from build123d import *

# Parameters (mm, degrees)
SKETCH_1_W                  = 325
SKETCH_1_H                  = 205
EXTRUDE_1_DEPTH             = 14
SKETCH_2_W                  = 7
SKETCH_2_H                  = 130
CUT_EXTRUDE_1_DEPTH         = 341.852240714
CUT_EXTRUDE_2_DEPTH         = 10
SKETCH_4_W                  = 3
SKETCH_4_H                  = 6
CUT_EXTRUDE_3_DEPTH         = 10
SKETCH_5_W                  = 3
SKETCH_5_H                  = 6
CUT_EXTRUDE_4_DEPTH         = 10
SKETCH_6_W                  = 315
SKETCH_6_H                  = 155
CUT_EXTRUDE_5_DEPTH         = 2
DRAFT_1_ANGLE               = 68.198590514
HOLE_WIZARD_3_5_3_5_1_D     = 3.5
HOLE_WIZARD_3_5_3_5_1_DEPTH = 5
FILLET_1_R                  = 1
FILLET_2_R                  = 2


with BuildPart() as part:
    # 草图1 → 凸台-拉伸1 (new body)
    with BuildSketch(Plane.XY.offset(7)):
        Rectangle(SKETCH_1_W, SKETCH_1_H)
    extrude(amount=-EXTRUDE_1_DEPTH)

    # 草图2 → 切除-拉伸1 (cut, through all)
    with BuildSketch(Plane(origin=(162.5, 0, 0), x_dir=(0, 0, -1), z_dir=(1, 0, 0))):
        with Locations((3.5, 37.5)):
            Rectangle(SKETCH_2_W, SKETCH_2_H)
    extrude(amount=-CUT_EXTRUDE_1_DEPTH, mode=Mode.SUBTRACT)

    # 草图3 → 切除-拉伸2 (cut)
    with BuildSketch(Plane(origin=(162.5, 0, 0), x_dir=(0, 0, -1), z_dir=(1, 0, 0))):
        Polygon((-2, -43.5), (0.946428571, -45), (2.946428571, -45), (2.946428571, -33), (0.946428571, -33), (-2, -34.5), align=None)
    extrude(amount=-CUT_EXTRUDE_2_DEPTH, mode=Mode.SUBTRACT)

    # 草图4 → 切除-拉伸3 (cut)
    with BuildSketch(Plane(origin=(162.5, 0, 0), x_dir=(0, 0, -1), z_dir=(1, 0, 0))):
        with Locations((-0.5, -60)):
            Rectangle(SKETCH_4_W, SKETCH_4_H)
    extrude(amount=-CUT_EXTRUDE_3_DEPTH, mode=Mode.SUBTRACT)

    # 草图5 → 切除-拉伸4 (cut)
    with BuildSketch(Plane(origin=(162.5, 0, 0), x_dir=(0, 0, -1), z_dir=(1, 0, 0))):
        with Locations((-0.5, -80)):
            Rectangle(SKETCH_5_W, SKETCH_5_H)
    extrude(amount=-CUT_EXTRUDE_4_DEPTH, mode=Mode.SUBTRACT)

    # 草图6 → 切除-拉伸5 (cut)
    with BuildSketch(Plane.XY.offset(7)):
        with Locations((0, 20)):
            Rectangle(SKETCH_6_W, SKETCH_6_H)
    extrude(amount=-CUT_EXTRUDE_5_DEPTH, mode=Mode.SUBTRACT)

    # 拔模1
    draft_1_faces = [part.faces().sort_by_distance(p)[0] for p in [
        (0, -27.5, -3.5),
    ]]
    draft(draft_1_faces, Plane(origin=(0, 0, -7), x_dir=(-1, 0, 0), z_dir=(0, 0, -1)), DRAFT_1_ANGLE)

    # Ø3.5 (3.5) 直径孔1
    with Locations(Plane(origin=(0, 0, -7), x_dir=(-1, 0, 0), z_dir=(0, 0, -1))):
        with Locations((-37.55, -37.75), (37.55, -37.75)):
            Hole(HOLE_WIZARD_3_5_3_5_1_D / 2, depth=HOLE_WIZARD_3_5_3_5_1_DEPTH)

    # 圆角1
    fillet_1_edges = [part.edges().sort_by_distance(p)[0] for p in [
        (-162.5, -65, -7),
        (162.5, 102.5, 3.5),
        (-162.5, 102.5, 3.5),
        (-162.5, -18.75, -3.5),
        (0, -27.5, -7),
        (-162.5, 46.25, 0),
        (0, -10, 0),
        (0, 102.5, 0),
        (162.5, 46.25, 0),
        (162.5, -18.75, -3.5),
        (0, -102.5, -7),
        (-162.5, 0, 7),
        (0, 102.5, 7),
        (162.5, 0, 7),
        (0, -102.5, 7),
        (-162.5, -102.5, 0),
        (162.5, -102.5, 0),
        (162.5, -65, -7),
    ]]
    fillet(fillet_1_edges, radius=FILLET_1_R)

    # 圆角2
    fillet_2_edges = [part.edges().sort_by_distance(p)[0] for p in [
        (-157.5, -57.5, 6),
        (-157.5, 97.5, 6),
        (157.5, 97.5, 6),
        (157.5, -57.5, 6),
    ]]
    fillet(fillet_2_edges, radius=FILLET_2_R)


solid = part.part
Input: part model. Units: mm. Frame: model coordinates. A direction names the side the tool comes from. Give positions to 0.01 mm unless a question says otherwise; leave off trailing zeros. Loops run counter-clockwise (first coordinate to the right, second up) from the corner with the lowest first, then second, coordinate; pieces in that order, holes last. Notation, with made-up numbers: (50.25, 69) -> (59.25, 69) arc R22 ccw to (59.25, 90) -> close; hole circle Ø8 at (10, 57.25). An arc over 180 degrees is marked (long way). Answer as a JSON object with one key per item and string values. Group by question number.
Item 1: Cut plane B-B, the plane y = 39.5. Return the cut outline in (x, z), and give its area (3 significant figures).
Item 2: Cut plane A-A, the plane x = -106. Return the cut outline in (y, z), and give its area (3 significant figures).
Item 3: Line query: probe 1 along Y at (x, z) = (-39.5, 5.25); probe 2 along Z at (x, y) = (-10.5, 72.5); probe 3 along Z at (x, y) = (94.5, -46.5). Output: solid intervals per line, ascending.
Item 4: Pull-direction query (Y, two-part tool) for faces 4 (the flat face through (-2, -102.5, 0)), 5 (the flat face through (2, 45, 0)), 6 (the flat face through (158, -80, -1)); classes: released by +Y, released by -Y, zero draft, split by the parting line, or undercut.
Item 5: Reachability of faces 1 (the flat face through (158, -60, 2)), 2 (the flat face through (-2, 21, 5)), 3 (the flat face through (-162.5, -24, 1)) from +Z, -Z, +X, -X, +Y, -Y: full face, straight path, thin tool, end or side. Return the list, or none.
Item 6: Pin query (flat end, axial travel): P1, Ø2, axis at x = 125, y = -7, coming from the -Z side; P2, Ø3, axis at x = 4.5, y = 6, coming from the +Z side; P3, Ø1.5, axis at x = -129, y = -21, coming from the -Z side. Return the tip coordinate at first contact, or that it passes through.
Checks:
{
 "1": {"outline": "(-162.5, 1) arc R1 ccw to (-161.5, 0) -> (161.5, 0) arc R1 ccw to (162.5, 1) -> (162.5, 6) arc R1 ccw to (161.5, 7) -> (157.5, 7) -> (157.5, 5) -> (-157.5, 5) -> (-157.5, 7) -> (-161.5, 7) arc R1 ccw to (-162.5, 6) -> close", "area": "1,640 mm²"},
 "2": {"outline": "(-102.5, -6) arc R1 ccw to (-101.5, -7) -> (-27.69, -7) arc R1 ccw to (-27.32, -6.93) -> (-10.18, -0.07) arc R1 cw to (-9.81, 0) -> (101.5, 0) arc R1 ccw to (102.5, 1) -> (102.5, 6) arc R1 ccw to (101.5, 7) -> (97.5, 7) -> (97.5, 5) -> (-57.5, 5) -> (-57.5, 7) -> (-101.5, 7) arc R1 ccw to (-102.5, 6) -> close", "area": "1,710 mm²"},
 "3": {"probe 1": "y = -102.5 to -57.5, 97.5 to 102.5", "probe 2": "z = 0 to 5", "probe 3": "z = -7 to 5"},
 "4": {"face 4": "released by -Y", "face 5": "zero draft", "face 6": "undercut"},
 "5": {"face 1": "+X", "face 2": "+Z", "face 3": "+Z, -Z, -X, +Y, -Y"},
 "6": {"P1": "stops at z = 0", "P2": "stops at z = 5", "P3": "stops at z = -4.7"}
}
